Model file for the job. Use its own axes, mm. A direction names the side the tool comes from. Coordinates: 2 decimals unless noted, no trailing zeros. Loops run counter-clockwise (first coordinate to the right, second up) from the corner with the lowest first, then second, coordinate; pieces in that order, holes last.
Autodesk Inventor part; units mm, degrees
ref_plane "Work Plane1" through (0, 0, 15) normal (0, 0, 1) x (1, 0, 0)
ref_plane "YZ Plane" through (0, 0, 0) normal (1, 0, 0) x (0, 1, 0)
ref_plane "XZ Plane" through (0, 0, 0) normal (0, 1, 0) x (-1, 0, 0)
sketch "Sketch1" plane through (0, 0, 0) normal (0, 0, 1) x (1, 0, 0)
  line L0 (10, 15) -> (-10, 15)
  line L1 (-15, 10) -> (-15, -15)
  line L2 (-15, -15) -> (15, -15)
  line L3 (15, -4) -> (15, 10)
  line L4 (15, 15) -> (-15, -15) construction
  line L5 (-15, 15) -> (15, -15) construction
  line L6 (15, -15) -> (55, -15)
  line L7 (85, -15) -> (85, -9)
  line L8 (-15, -9) -> (-15, -15)
  line L9 (85, -15) -> (55, -15)
  line L10 (55, -4) -> (55, 10)
  line L11 (60, 15) -> (80, 15)
  line L12 (85, 10) -> (85, -15)
  line L13 (50, -9) -> (20, -9)
  arc A0 (-10, 15) -> (-15, 10) centre (-10, 10) ccw
  arc A1 (15, 10) -> (10, 15) centre (10, 10) ccw
  arc A2 (15, -4) -> (20, -9) centre (20, -4) ccw
  arc A3 (50, -9) -> (55, -4) centre (50, -4) ccw
  arc A4 (60, 15) -> (55, 10) centre (60, 10) ccw
  arc A5 (85, 10) -> (80, 15) centre (80, 10) ccw
  point P0 (0, 0)
  point P1 (55, 15)
  point P2 (85, 15)
  dimension "d0" = 30
  dimension "d1" = 30
  dimension "d2" = 100
  dimension "d3" = 6
  dimension "d4" = 30
  dimension "d5" = 30
  dimension "d6" = 5
extrude "Extrusion1" add sketch "Sketch1" along normal blind 10
ref_plane "Work Plane1" through (0, 0, 15) normal (0, 0, 1) x (1, 0, 0)
mirror "Mirror1" about plane through (0, 0, 15) normal (0, 0, 1)
sketch "Sketch3" plane through (0, 0, 10) normal (0, 0, 1) x (1, 0, 0)
  line L0 (-15, -15) -> (85, -15)
  line L1 (85, -15) -> (85, -9)
  line L2 (85, -9) -> (-15, -9)
  line L3 (-15, -9) -> (-15, -15)
  point P0 (0, 0)
  dimension "d14" = 100
  dimension "d15" = 6
extrude "Extrusion3" add sketch "Sketch3" along normal blind 10
sketch "Sketch4" plane through (0, 0, 0) normal (0, 0, -1) x (-1, 0, 0)
  line L0 (-60, 15) -> (-80, 15)
  line L1 (-55, -4) -> (-55, 10)
  line L2 (-85, -15) -> (15, -15)
  line L3 (-35, -15) -> (-35, -9)
  line L4 (-20, -9) -> (-50, -9)
  point P0 (0, 0)
  point P1 (-70, 3)
  point P2 (0, 3)
  dimension "d18" = 12
  dimension "d19" = 15
hole "Hole1" at (70, 3, 0) at (0, 3, 0) direction (0, 0, 1) diameter 9 end through all
sketch "Sketch5" plane through (0, 0, 0) normal (0, 0, -1) x (-1, 0, 0)
  circle A0 centre (-70, 3) radius 4.5
  line L0 (-66, 9.9282) -> (-62, 3)
  line L1 (-62, 3) -> (-66, -3.9282)
  line L2 (-66, -3.9282) -> (-74, -3.9282)
  line L3 (-74, -3.9282) -> (-78, 3)
  line L4 (-78, 3) -> (-74, 9.9282)
  line L5 (-74, 9.9282) -> (-66, 9.9282)
  line L6 (-70, 3) -> (-55, 3)
  line L7 (-55, 10) -> (-55, -4)
  line L8 (-85, -15) -> (15, -15)
  line L9 (-35, -15) -> (-35, -9)
  line L10 (-20, -9) -> (-50, -9)
  line L11 (-4, 9.9282) -> (-8, 3)
  line L12 (-8, 3) -> (-4, -3.9282)
  line L13 (-4, -3.9282) -> (4, -3.9282)
  line L14 (4, -3.9282) -> (8, 3)
  line L15 (8, 3) -> (4, 9.9282)
  line L16 (4, 9.9282) -> (-4, 9.9282)
  circle A1 centre (0, 3) radius 4.5
  point P0 (0, 0)
  dimension "d27" = 16
extrude "Extrusion4" cut sketch "Sketch5" against normal blind 7
sketch "Sketch6" plane through (-15, -15, 30) normal (0, 0, 1) x (1, 0, 0)
  circle A0 centre (15, 18) radius 4.5
  line L0 (19, 11.0718) -> (23, 18)
  line L1 (19, 11.0718) -> (11, 11.0718)
  line L2 (11, 11.0718) -> (7, 18)
  line L3 (7, 18) -> (11, 24.9282)
  line L4 (11, 24.9282) -> (19, 24.9282)
  line L5 (19, 24.9282) -> (23, 18)
  line L6 (23, 18) -> (19, 11.0718)
  circle A1 centre (85, 18) radius 4.5
  line L7 (81, 11.0718) -> (89, 11.0718)
  line L8 (89, 11.0718) -> (81, 11.0718)
  line L9 (81, 11.0718) -> (77, 18)
  line L10 (77, 18) -> (81, 24.9282)
  line L11 (81, 24.9282) -> (89, 24.9282)
  line L12 (89, 24.9282) -> (93, 18)
  line L13 (93, 18) -> (89, 11.0718)
  point P0 (15, 15)
extrude "Extrusion5" cut sketch "Sketch6" against normal blind 7
properties part number "Suporte Carretel"
Q1. Which spindle directions (+Z, -Z, +X, -X, +Y, -Y) get a long thin tool onto all of the face, cutting with end or side? Do faces 5 (the flat face through (-6.028, 6.416, 3.451)), 6 (the flat face through (15, 3, 25)), 7 (the flat face through (76.028, -0.416, 26.549)). Say none if no direction does.
Answers:
face 5: -Z
face 6: +Z, -Z, +Y
face 7: +Z
Q2. Drill centre lines: line 1 (X direction, y = 3, z = 20.8); line 2 (Z direction, x = 6.5, y = 0.5); line 3 (Z direction, x = 78, y = -8.75). Where is each one in solid material? Low to high.
Answers:
line 1: x = -15 to -4.5, 4.5 to 15, 55 to 65.5, 74.5 to 85
line 2: z = 7 to 10, 20 to 23
line 3: z = 0 to 10, 20 to 30
Q3. Slice it at D-D (z = 12.75). List the corners of the cut face in (x, y), and give its area (3 significant figures).
Answers:
outline: (-15, -15) - (85, -15) - (85, -9) - (-15, -9) - close
area: 600 mm2
Q4. Slice it at A-A (z = 5.75). List the corners of the cut face in (x, y), and give its area (3 significant figures).
Answers:
outline: (-15, -15) - (85, -15) - (85, 10) arc R5 ccw to (80, 15) - (60, 15) arc R5 ccw to (55, 10) - (55, -4) arc R5 cw to (50, -9) - (20, -9) arc R5 cw to (15, -4) - (15, 10) arc R5 ccw to (10, 15) - (-10, 15) arc R5 ccw to (-15, 10) - close; hole (-8, 3) - (-4, -3.93) - (4, -3.93) - (8, 3) - (4, 9.93) - (-4, 9.93) - close; hole (62, 3) - (66, -3.93) - (74, -3.93) - (78, 3) - (74, 9.93) - (66, 9.93) - close
area: 1,700 mm2
Q5. Flat gauge pins, fed straight in: P1, Ø10.5, axis at x = 70, y = 3, coming from the +Z side; P2, Ø15, axis at x = 38.5, z = 13.5, coming from the +Y side; P3, Ø10.5, axis at x = 0, y = 3, coming from the -Z side. Where does each tip first touch, or does it go through?
Answers:
P1: stops at z = 23
P2: stops at y = -9
P3: stops at z = 7
Q6. Mould opens along X. For faces 1 (the flat face through (66.6, 6.2, 7)), 2 (the cylindrical face through (13, 14, 5)), 3 (the cylindrical face through (-13, 14, 25)), 4 (the flat face through (0, 15, 25)) say: +X half, -X half, draft (parallel to the pull), parting line (faces both ways), or undercut.
Answers:
face 1: undercut
face 2: undercut
face 3: -X half
face 4: draft
Q7. Slice it at C-C (y = -5.25). List the corners of the cut face in (x, z).
Answers:
outline: (-15, 0) - (15.16, 0) - (15.16, 10) - (-15, 10) - close; (-15, 20) - (15.16, 20) - (15.16, 30) - (-15, 30) - close; (54.84, 0) - (85, 0) - (85, 10) - (54.84, 10) - close; (54.84, 20) - (85, 20) - (85, 30) - (54.84, 30) - close
Q8. Slice it at B-B (x = 0). List the corners of the cut face in (y, z).
Answers:
outline: (-15, 0) - (-3.93, 0) - (-3.93, 7) - (-1.5, 7) - (-1.5, 10) - (-9, 10) - (-9, 20) - (-1.5, 20) - (-1.5, 23) - (-3.93, 23) - (-3.93, 30) - (-15, 30) - close; (7.5, 7) - (9.93, 7) - (9.93, 0) - (15, 0) - (15, 10) - (7.5, 10) - close; (7.5, 20) - (15, 20) - (15, 30) - (9.93, 30) - (9.93, 23) - (7.5, 23) - close
